Part model, mm, in its own coordinate system. A direction names the side the tool comes from. Coordinates: 2 decimals unless noted, no trailing zeros. Write each loop counter-clockwise with the first axis right and the second up, starting at its lowest first coordinate (ties: lowest second). Pieces come first, ordered by that corner, then holes. Notation, with made-up numbers: (4, 15.5) - (60, 15.5) arc R25 ccw to (60, 51.5) - close; hole circle Ø7 at (-14.5, 71). An arc over 180 degrees is marked (long way). Use a Markdown table: item, result.
```python
from build123d import *

# Parameters (mm, degrees)
F0_W     = 25.4
F0_H     = 25.4
F1_DEPTH = 50.8
F2_DEPTH = 25.4


with BuildPart() as f1:
    # F0 (on Front) → F1 (new body)
    with BuildSketch(Plane.XZ):
        with Locations((-12.7, 12.7)):
            Rectangle(F0_W, F0_H)
    extrude(amount=F1_DEPTH)

    # F0 (on Front) → F2 (join)
    with BuildSketch(Plane.XZ):
        with Locations((12.7, 38.1)):
            Rectangle(F0_W, F0_H)
        with Locations((12.7, 12.7)):
            Rectangle(F0_W, F0_H)
    extrude(amount=F2_DEPTH)


solid = f1.part
```
Item 1: Drop flat-ended pins along their axis: P1, Ø5, axis at x = 14.5, z = 10.5, coming from the -Y side; P2, Ø4, axis at x = -14, y = -32, coming from the +Z side; P3, Ø20.5, axis at y = -40.5, z = 13.5, coming from the +X side. Give the stop position or say it passes through.
From the geometry:
| item | result |
|---|---|
| P1 | y = -25.4 |
| P2 | z = 25.4 |
| P3 | x = 0 |
Item 2: Which spindle directions (+Z, -Z, +X, -X, +Y, -Y) get a long thin tool onto all of the face, cutting with end or side? Do faces 1 (the face through (13, -25.4, 26)), 2 (the face through (5, 0, 20)), 3 (the face through (0, -13, 38)). Say none if no direction does.
From the geometry:
| item | result |
|---|---|
| face 1 | +Z, -Z, +X, -Y |
| face 2 | +Z, -Z, +X, -X, +Y |
| face 3 | +Z, -X, +Y, -Y |
Item 3: Band-saw the part on A-A, the plane z = 6. Give the cut face in (x, y).
From the geometry:
| item | result |
|---|---|
| outline | (-25.4, -50.8) - (0, -50.8) - (0, -25.4) - (25.4, -25.4) - (25.4, 0) - (-25.4, 0) - close |
Item 4: Band-saw the part on B-B, the plane y = -37. Give the cut face in (x, z).
From the geometry:
| item | result |
|---|---|
| outline | (-25.4, 0) - (0, 0) - (0, 25.4) - (-25.4, 25.4) - close |
Item 5: Band-saw the part on C-C, the plane x = 7.5. Give the cut face in (y, z), then the cut area to 3 significant figures.
From the geometry:
| item | result |
|---|---|
| outline | (-25.4, 0) - (0, 0) - (0, 50.8) - (-25.4, 50.8) - close |
| area | 1,290 mm^2 |
Item 6: Band-saw the part on D-D, the plane y = -19.5. Give the cut face in (x, z), then the cut area to 3 significant figures.
From the geometry:
| item | result |
|---|---|
| outline | (-25.4, 0) - (25.4, 0) - (25.4, 50.8) - (0, 50.8) - (0, 25.4) - (-25.4, 25.4) - close |
| area | 1,940 mm^2 |
Item 7: Drill centre lines: probe 1 along Y at (x, z) = (20, 7); probe 2 along Z at (x, y) = (-5.5, -6.5). Where is each one in solid material? Low to high.
From the geometry:
| item | result |
|---|---|
| probe 1 | -25.4 to 0 |
| probe 2 | 0 to 25.4 |
